from build123d import *

# Parameters (mm, degrees)
SKETCH_1_W          = 40
SKETCH_1_H          = 20
EXTRUDE_1_DEPTH     = 6
SKETCH_2_R          = 2.5
CUT_EXTRUDE_1_DEPTH = 24.151673806
EXTRUDE_START       = -15
EXTRUDE_2_OUTLINE_R = 11
EXTRUDE_2_DEPTH     = 15
EXTRUDE_START_2     = -8
SKETCH_5_R          = 11
SKETCH_5_R_2        = 10
EXTRUDE_3_DEPTH     = 8
SKETCH_10_W         = 15
SKETCH_10_H         = 5
EXTRUDE_4_DEPTH     = 200
SKETCH_11_W         = 3.09493726
SKETCH_11_H         = 3.09493726
EXTRUDE_5_DEPTH     = 15
SKETCH_17_W         = 83.501719846
SKETCH_17_H         = 42.356909186
CUT_EXTRUDE_2_DEPTH = 184.131783151
SKETCH_18_R         = 2.5
CUT_EXTRUDE_3_DEPTH = 10
SKETCH_20_R         = 2.837069856
CUT_EXTRUDE_4_DEPTH = 10


# Read off the part's stored shape, not the designer's step: 凸台-拉伸2
with BuildPart() as part:
    # 草图1 → 凸台-拉伸1 (new body)
    with BuildSketch(Plane.XY):
        Rectangle(SKETCH_1_W, SKETCH_1_H)
    extrude(amount=EXTRUDE_1_DEPTH)

    # 草图2 → 切除-拉伸1 (cut, through all)
    with BuildSketch(Plane.XY.offset(6)):
        with Locations((10, 0)):
            Circle(SKETCH_2_R)
        with Locations((-1, 0)):
            Circle(SKETCH_2_R)
        with Locations((-12, 0)):
            Circle(SKETCH_2_R)
    extrude(amount=-CUT_EXTRUDE_1_DEPTH, mode=Mode.SUBTRACT)

    # 凸台-拉伸2 outline → 凸台-拉伸2 (add)
    with BuildSketch(Plane.XY.offset(6).offset(EXTRUDE_START)):
        with BuildLine():
            Line((20, 10), (20, 13.5))
            Line((20, 13.5), (-26.893967141, 13.5))
            Line((-26.893967141, 13.5), (-26.893967141, 13.384337644))
            ThreePointArc((-26.893967141, 13.384337644), (-45, 0), (-26.893967141, -13.384337644))
            Line((-26.893967141, -13.384337644), (-26.893967141, -13.5))
            Line((-26.893967141, -13.5), (20, -13.5))
            Line((20, -13.5), (20, -10))
            Line((20, -10), (-20, -10))
            Line((-20, -10), (-20, -8.660254038))
            ThreePointArc((-20, -8.660254038), (-17, 0), (-20, 8.660254038))
            Line((-20, 8.660254038), (-20, 10))
            Line((-20, 10), (20, 10))
        make_face()
        with Locations((-31, 0)):
            Circle(EXTRUDE_2_OUTLINE_R, mode=Mode.SUBTRACT)
    extrude(amount=EXTRUDE_2_DEPTH)

    # 草图5 → 凸台-拉伸3 (add)
    with BuildSketch(Plane.XY.offset(6).offset(EXTRUDE_START_2)):
        with Locations((-31, 0)):
            Circle(SKETCH_5_R)
        with Locations((-31, 0)):
            Circle(SKETCH_5_R_2, mode=Mode.SUBTRACT)
    extrude(amount=EXTRUDE_3_DEPTH)

    # 草图10 → 凸台-拉伸4 (add)
    with BuildSketch(Plane(origin=(20, 0, 0), x_dir=(0, 0, -1), z_dir=(1, 0, 0))):
        with Locations((1.5, -16)):
            Rectangle(SKETCH_10_W, SKETCH_10_H)
    extrude(amount=-EXTRUDE_4_DEPTH)

    # 草图11 → 凸台-拉伸5 (add, through all)
    with BuildSketch(Plane.XY.offset(6)):
        with Locations((-27.071814196, -13.413570993)):
            Rectangle(SKETCH_11_W, SKETCH_11_H)
    extrude(amount=-EXTRUDE_5_DEPTH)

    # 草图17 → 切除-拉伸2 (cut, through all)
    with BuildSketch(Plane.XZ.offset(18.5)):
        with Locations((-150.158557574, 4.061352957)):
            Rectangle(SKETCH_17_W, SKETCH_17_H)
    extrude(amount=-CUT_EXTRUDE_2_DEPTH, mode=Mode.SUBTRACT)

    # 草图18 → 切除-拉伸3 (cut)
    with BuildSketch(Plane.XZ.offset(18.5)):
        with Locations(Location((-98.407697651, -1.5, 0), (0, 0, 270))):
            Circle(SKETCH_18_R)
    extrude(amount=-CUT_EXTRUDE_3_DEPTH, mode=Mode.SUBTRACT)

    # 草图20 → 切除-拉伸4 (cut)
    with BuildSketch(Plane.XZ.offset(18.5)):
        with Locations(Location((-54.23606844, 0.343836832, 0), (0, 0, 270))):
            Circle(SKETCH_20_R)
        with Locations(Location((-80.23606844, 0.343836832, 0), (0, 0, 270))):
            Circle(SKETCH_20_R)
    extrude(amount=-CUT_EXTRUDE_4_DEPTH, mode=Mode.SUBTRACT)


solid = part.part
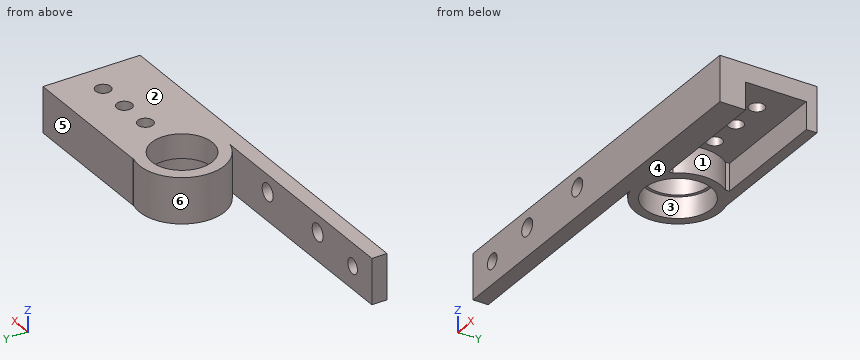
CAD build for the part. Positions are in the model's coordinates, mm. Face numbers are marked on the shaded views. A direction names the side the tool comes from. Give positions to 0.01 mm unless a question says otherwise; leave off trailing zeros. Order: outer loops, then holes, each group sorted by start corner. A loop starts at its lowest first (then second) coordinate and runs counter-clockwise, first axis right, second up. Notation, with made-up numbers: (44, -28.5) - (56, -28.5) arc R23 cw to (56, -16.5) - close; hole circle Ø5 at (61.25, 55.5). An arc over 180 degrees is marked (long way). Write each question's results on one line, items separated by ' | '.
1. Pull direction Y, two halves, no side cores. Call the marked faces 4, 5 and 6: released by +Y, released by -Y, zero draft, split by the parting line, or undercut.
Calculated:
face 4: zero draft | face 5: released by +Y | face 6: undercut
2. 3-axis set-ups, long thin cutter, end or side, ignore diameter. For the marked faces 1, 2 and 3: which of +Z, -Z, +X, -X, +Y, -Y reach the whole face in a straight line?
Calculated:
face 1: -Z, +X | face 2: +Z, +X, -X, +Y, -Y | face 3: -Z
3. Probe L1, parallel to Y at x = -31, z = 3.75; L2, parallel to Y at x = -31, z = -4.25; L3, parallel to Y at x = -100.5, z = 4.5. List the from-to ranges inside material, lowest first. Write a range as from..to.
Calculated:
L1: y = -18.5..-10, 10..14 | L2: y = -18.5..-11, 11..14 | L3: y = -18.5..-13.5
4. Pin check, flat tips, straight feed: pin 1 (9 mm diameter, centred on x = -54.24, z = 0.34, fed in from +Y); pin 2 (4.5 mm diameter, centred on x = -98.41, z = -1.5, fed in from -Y); pin 3 (4.5 mm diameter, centred on x = 3, z = -2.5, fed in from +Y); pin 4 (1 mm diameter, centred on y = -1.5, z = -6, fed in from +X). Stop position of each tip, or through.
Calculated:
pin 1: stops at y = -13.5 | pin 2: passes through | pin 3: stops at y = 13.5 | pin 4: stops at x = -17.04
5. Saw through at C-C on x = 10. List the corners of the cut face in (y, z).
Calculated:
outline: (-18.5, -9) - (-10, -9) - (-10, 0) - (-2.5, 0) - (-2.5, 6) - (-18.5, 6) - close; (2.5, 0) - (10, 0) - (10, -9) - (13.5, -9) - (13.5, 6) - (2.5, 6) - close
6. Saw through at B-B on y = 0. List the corners of the cut face in (x, z), and give its area (3 significant figures).
Calculated:
outline: (-45, -9) - (-42, -9) - (-42, -2) - (-41, -2) - (-41, 6) - (-45, 6) - close; (-21, -2) - (-20, -2) - (-20, -9) - (-17, -9) - (-17, 0) - (-14.5, 0) - (-14.5, 6) - (-21, 6) - close; (-9.5, 0) - (-3.5, 0) - (-3.5, 6) - (-9.5, 6) - close; (1.5, 0) - (7.5, 0) - (7.5, 6) - (1.5, 6) - close; (12.5, 0) - (20, 0) - (20, 6) - (12.5, 6) - close | area: 238 mm2
7. Saw through at A-A on x = -31. List the corners of the cut face in (y, z), and give its area (4 significant figures).
Calculated:
outline: (-18.5, -9) - (-11, -9) - (-11, -2) - (-10, -2) - (-10, 6) - (-18.5, 6) - close; (10, -2) - (11, -2) - (11, -9) - (14, -9) - (14, 6) - (10, 6) - close | area: 173.5 mm2
8. Saw through at D-D on x = -68. List the corners of the cut face in (y, z), and give its area (3 significant figures).
Calculated:
outline: (-18.5, -9) - (-13.5, -9) - (-13.5, 6) - (-18.5, 6) - close | area: 75.0 mm2
